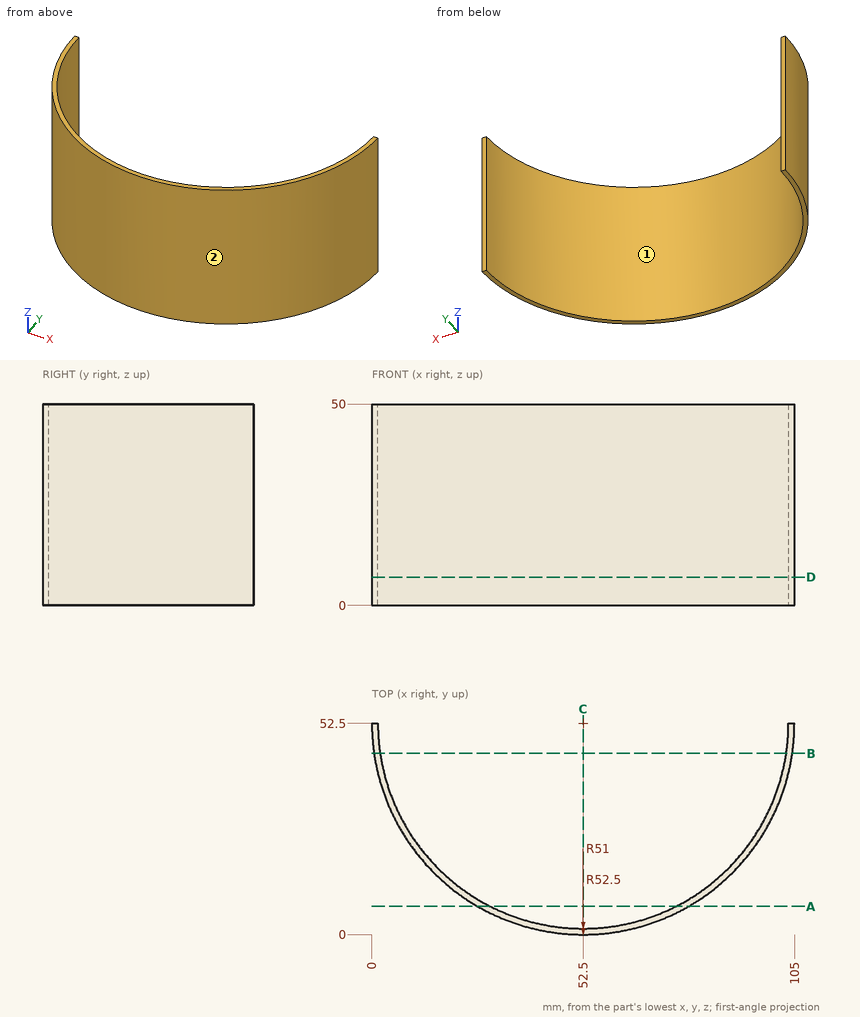
The figure shows three views and two pictorial views of one solid part (mm, origin at its lowest corner). Answer the questions. Coordinates: 2 decimals unless noted, no trailing zeros. Loops run counter-clockwise (first coordinate to the right, second up) from the corner with the lowest first, then second, coordinate; pieces in that order, holes last. Notation, with made-up numbers: M 51,15.25 L 64,15.25 A38 cw 64,54.25 Z; hole C 78.25,86.25 d1. An arc over 180 degrees is marked long. Use CSV: the item, a comma, the result in double quotes. Start each with the question number.
(1) Find section C-C, the plane x = 52.5. Give the vertices of the cut face in (y, z).
(2) Given pin 1 Ø6 at (x, z) = (58.5, 29.5) entering from -Y; pin 2 Ø12 at (y, z) = (10, 40.5) entering from +X; pin 3 Ø6 at (x, z) = (75, 18) entering from -Y, each flat-ended and moving along its own axis, determine where each tip first touches the part or whether it passes through.
(3) Find section D-D, the plane z = 7. Give the vertices of the cut face in (x, y).
(4) Find section A-A, the plane y = 7. Give the vertices of the cut face in (x, z), then the cut area to 3 significant figures.
(5) Consider line 1 (X direction, y = 49.5, z = 25); line 2 (X direction, y = 24, z = 3.5); line 3 (Y direction, x = 52, z = 43). Determine where each line is inside the solid, lowest interval first.
(6) For a pull along X with two mould halves and no side action, classify the marked faces 1 and 2 as +X half, -X half, draft (parallel to the pull), parting line (faces both ways), or undercut.
(7) Find section B-B, the plane y = 45. Give the vertices of the cut face in (x, z).
Recorded:
1,outline,"M 0,0 L 1.5,0 L 1.5,50 L 0,50 Z"
2,pin 1,"stops at y = 0.09"
2,pin 2,"stops at x = 90.24"
2,pin 3,"stops at y = 3.76"
3,outline,"M 0,52.5 A52.5 ccw 105,52.5 L 103.5,52.5 A51 cw 1.5,52.5 Z"
4,outline,"M 26.31,0 L 29.46,0 L 29.46,50 L 26.31,50 Z; M 75.54,0 L 78.69,0 L 78.69,50 L 75.54,50 Z"
4,area,"315 mm^2"
5,line 1,"x = 0.09 to 1.59, 103.41 to 104.91"
5,line 2,"x = 8.41 to 10.21, 94.79 to 96.59"
5,line 3,"y = 0 to 1.5"
6,face 1,"undercut"
6,face 2,"parting line"
7,outline,"M 0.54,0 L 2.05,0 L 2.05,50 L 0.54,50 Z; M 102.95,0 L 104.46,0 L 104.46,50 L 102.95,50 Z"
